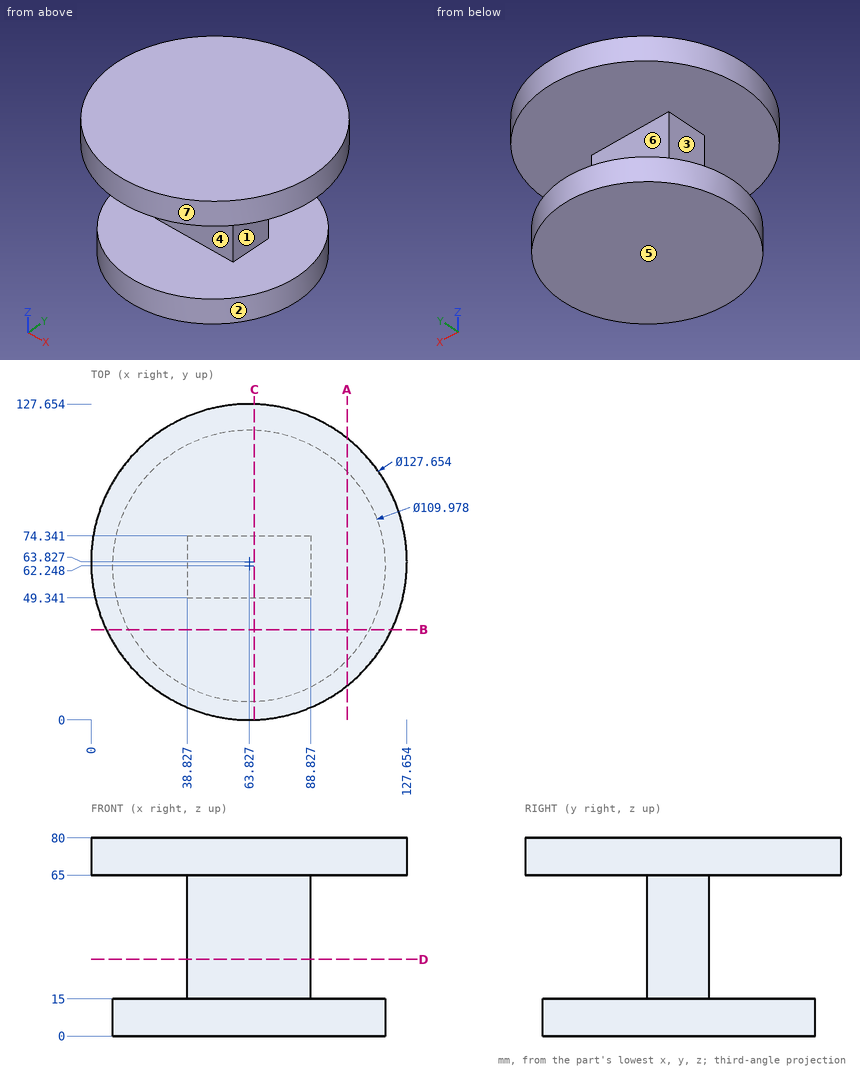
Design review of the part shown in the three views and the two pictorial views. Dimensions are in mm from the part's minimum x, y and z. A direction names the side the tool comes from. Round coordinates to 2 decimals unless told otherwise and drop trailing zeros. Loops run counter-clockwise (first coordinate to the right, second up) from the corner with the lowest first, then second, coordinate; pieces in that order, holes last. Notation, with made-up numbers: (44, 19) -> (53, 19) arc R21 cw to (53, 47) -> close; hole circle Ø1 at (17.5, -27). An arc over 180 degrees is marked (long way). Answer as CSV lines item,"result".
1) Add section B-B on y = 36.5. Write out the cut boundary in (x, z) (1 decimal).
Geometry results:
outline,"(6.1, 65) -> (121.5, 65) -> (121.5, 80) -> (6.1, 80) -> close; (15.2, 0) -> (112.4, 0) -> (112.4, 15) -> (15.2, 15) -> close"
2) Add section D-D on z = 31. Write out the cut boundary in (x, y).
Geometry results:
outline,"(38.83, 49.34) -> (88.83, 49.34) -> (88.83, 74.34) -> (38.83, 74.34) -> close"
3) Draft analysis for pull direction Z (two halves, no side actions). For the marked faces 5, 6 and 7, state which applies: pulls with the +Z half, pulls with the -Z half, needs draft (parallel to the pull), parting line crosses it, or undercut.
Geometry results:
face 5,"pulls with the -Z half"
face 6,"undercut"
face 7,"needs draft"
4) Tool access review of the marked faces 1, 2, 3 and 4: name each direction out of +Z, -Z, +X, -X, +Y, -Y from which nothing blocks a thin tool from reaching the whole face with its end or side.
Geometry results:
face 1,"+X, +Y, -Y"
face 2,"-Z"
face 3,"-X, +Y, -Y"
face 4,"+X, -X, -Y"
5) To check wall thickness, follow line 1 along Z through (x, y) = (85, 75.5); line 2 along Z through (x, y) = (28, 111); line 3 along X through (y, z) = (72, 45.5). State the ranges of each line that lie inside material, in increasing order. Write a range as from..to.
Geometry results:
line 1,"z = 0..15, 65..80"
line 2,"z = 65..80"
line 3,"x = 38.83..88.83"
6) Add section A-A on x = 103.5. Write out the cut boundary in (y, z) (1 decimal).
Geometry results:
outline,"(13.8, 65) -> (113.8, 65) -> (113.8, 80) -> (13.8, 80) -> close; (24.2, 0) -> (100.3, 0) -> (100.3, 15) -> (24.2, 15) -> close"
7) Add section C-C on x = 66. Write out the cut boundary in (y, z).
Geometry results:
outline,"(0.04, 65) -> (49.34, 65) -> (49.34, 15) -> (7.3, 15) -> (7.3, 0) -> (117.19, 0) -> (117.19, 15) -> (74.34, 15) -> (74.34, 65) -> (127.62, 65) -> (127.62, 80) -> (0.04, 80) -> close"
8) For P1, Ø10, axis at x = 83, z = 35.5, coming from the -Y side; P2, Ø8, axis at y = 73, z = 69.5, coming from the +X side; P3, Ø6, axis at y = 59, z = 65, coming from the -X side, all flat-tipped, find the tip position at first contact; note any pin that passes through.
Geometry results:
P1,"stops at y = 49.34"
P2,"stops at x = 127.44"
P3,"stops at x = 0.03"
